Study the drawing (mm; zero at the part's minimum x, y, z) and answer. Coordinates: 2 decimals unless noted, no trailing zeros. Order: outer loops, then holes, each group sorted by start corner. A loop starts at its lowest first (then second) coordinate and runs counter-clockwise, first axis right, second up.
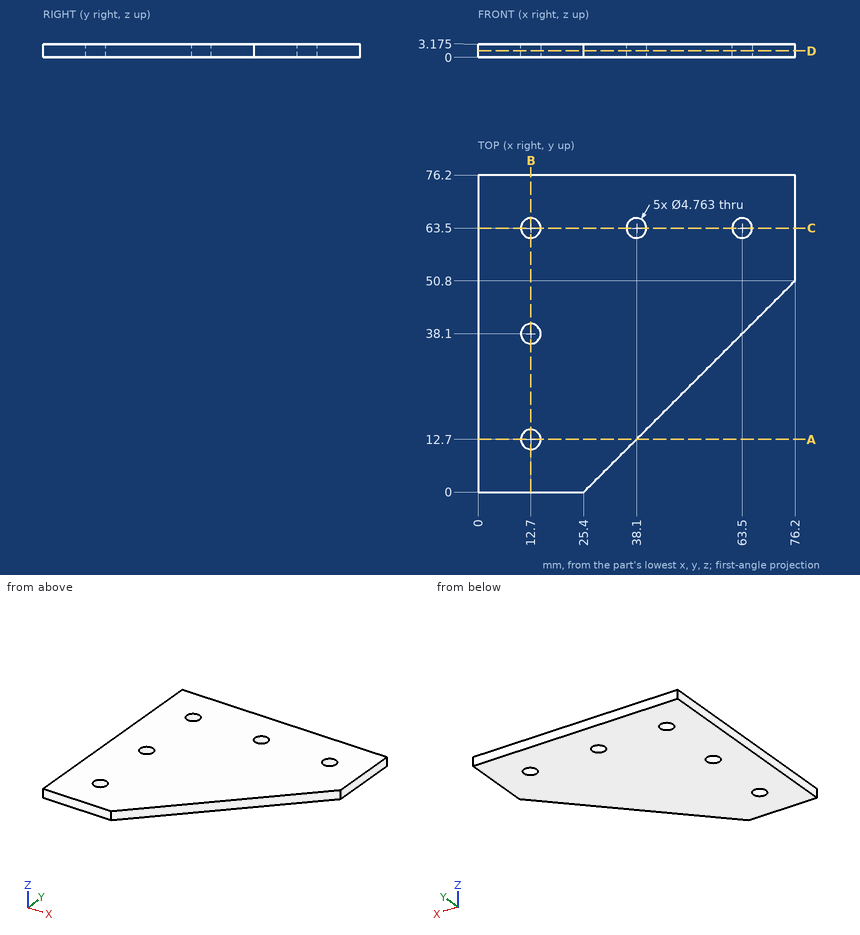
1) A cutting plane is placed at B-B, the plane x = 12.7. Determine the outline of the cut face in (y, z) (1 decimal).
A:
outline: (0, 0) - (10.3, 0) - (10.3, 3.2) - (0, 3.2) - close; (15.1, 0) - (35.7, 0) - (35.7, 3.2) - (15.1, 3.2) - close; (40.5, 0) - (61.1, 0) - (61.1, 3.2) - (40.5, 3.2) - close; (65.9, 0) - (76.2, 0) - (76.2, 3.2) - (65.9, 3.2) - close
2) Flat-ended cylindrical pins translate along their axes: pin 1 Ø7.5 at (x, y) = (12.7, 12.7) entering from +Z (3 decimals); pin 2 Ø1.5 at (y, z) = (17, 0.5) entering from +X. Find the tip coordinate at first contact, or state that the pin passes through.
A:
pin 1: stops at z = 3.175
pin 2: stops at x = 43.15
3) A cutting plane is placed at A-A, the plane y = 12.7. Determine the outline of the cut face in (x, z) (1 decimal).
A:
outline: (0, 0) - (10.3, 0) - (10.3, 3.2) - (0, 3.2) - close; (15.1, 0) - (38.1, 0) - (38.1, 3.2) - (15.1, 3.2) - close
4) Straight lines are drawn through the part: line 1 (Y direction, x = 12.7, z = 1.8); line 2 (X direction, y = 37, z = 2.8); line 3 (X direction, y = 18, z = 2.25). For each, find the intervals that lie inside material, in ascending order.
A:
line 1: y = 0 to 10.32, 15.08 to 35.72, 40.48 to 61.12, 65.88 to 76.2
line 2: x = 0 to 10.59, 14.81 to 62.4
line 3: x = 0 to 43.4
5) A cutting plane is placed at D-D, the plane z = 1.55. Determine the outline of the cut face in (x, y).
A:
outline: (0, 0) - (25.4, 0) - (76.2, 50.8) - (76.2, 76.2) - (0, 76.2) - close; hole circle Ø4.76 at (12.7, 12.7); hole circle Ø4.76 at (12.7, 38.1); hole circle Ø4.76 at (12.7, 63.5); hole circle Ø4.76 at (38.1, 63.5); hole circle Ø4.76 at (63.5, 63.5)
